Design review of the part built by this model. Coordinates are the model's own, in mm. A direction names the side the tool comes from. Coordinates: 2 decimals unless noted, no trailing zeros. Write each loop counter-clockwise with the first axis right and the second up, starting at its lowest first coordinate (ties: lowest second). Pieces come first, ordered by that corner, then holes.
Q1. Insertion check: pin 1 (3 mm diameter, centred on x = -8, z = 9, fed in from +Y); pin 2 (1.5 mm diameter, centred on x = 12, z = 9, fed in from -Y); pin 3 (3.5 mm diameter, centred on x = 3, z = 4.5, fed in from +Y). Each pin has a flat end and moves straight along its axis. Give the tip position at first contact, or say it passes through.
Q2. Machinability: for faces 5 (the flat face through (15, 10, 6)), 6 (the flat face through (0, -11, 6)), which of the approach directions +Z, -Z, +X, -X, +Y, -Y give a long, thin tool a straight path to every point of the face, cutting with its end or side? Answer none if there is none.
Q3. Take a section at C-C (z = 7.75). Give the boundary of the cut face in (x, y) (3 decimals), and give its area (3 significant figures).
Q4. Take a section at B-B (y = 14). Give the boundary of the cut face in (x, z).
Q5. Take a section at A-A (x = 0). Give the boundary of the cut face in (y, z) (3 decimals), and give its area (3 significant figures).
Q6. For probe 1 along Y at (x, z) = (0, 7.5) (3 decimals); probe 2 along X at (y, z) = (6, 5.5); probe 3 along X at (y, z) = (24, 2.75), list the stretches that pass through material, from the lowest coordinate up.
Q7. Mouldability with a two-part tool opening along Y and no side actions: class faces 1 (the flat face through (0, 11, 0)), 2 (the flat face through (-8.718, -2, 6)), 3 (the cylindrical face through (0, -40, 6)), 4 (the flat face through (0, 7, 6)) as pulls with the +Y half, pulls with the -Y half, needs draft (parallel to the pull), parting line crosses it, or undercut.
Q8. Take a section at D-D (x = 13.5). Give the boundary of the cut face in (y, z), and give its area (3 significant figures).
```python
from build123d import *

# Parameters (mm, degrees)
SKETCH1_R           = 9.625
SKETCH1_R_2         = 5
SKETCH1_W           = 18
SKETCH1_H           = 18
BOSS_EXTRUDE1_DEPTH = 12


with BuildPart() as part:
    # Sketch1 → Boss-Extrude1 (new body)
    with BuildSketch(Plane.XY):
        with BuildLine():
            Line((15, 45), (15, -25))
            ThreePointArc((15, -25), (0, -40), (-15, -25))
            Line((-15, -25), (-15, 45))
            ThreePointArc((-15, 45), (0, 60), (15, 45))
        make_face()
        with Locations((0, -25)):
            Circle(SKETCH1_R, mode=Mode.SUBTRACT)
        with Locations((0, 45)):
            Circle(SKETCH1_R_2, mode=Mode.SUBTRACT)
        with Locations((0, 21)):
            Rectangle(SKETCH1_W, SKETCH1_H, mode=Mode.SUBTRACT)
        with Locations((0.28234497, -2)):
            Rectangle(SKETCH1_W, SKETCH1_H, mode=Mode.SUBTRACT)
    extrude(amount=BOSS_EXTRUDE1_DEPTH)


solid = part.part
```
Response:
1. pin 1: stops at y = 58.52
1. pin 2: stops at y = -34.92
1. pin 3: stops at y = 59.95
2. face 5: +Z, -Z, +X, +Y, -Y
2. face 6: +Z, -Z
3. outline: (-15, -25) arc R15 ccw to (15, -25) - (15, 45) arc R15 ccw to (-15, 45) - close; hole circle Ø19.25 at (0, -25); hole (-9, 12) - (9, 12) - (9, 30) - (-9, 30) - close; hole (-8.718, -11) - (9.282, -11) - (9.282, 7) - (-8.718, 7) - close; hole circle Ø10 at (0, 45)
3. area: 1,790 mm2
4. outline: (-15, 0) - (-9, 0) - (-9, 12) - (-15, 12) - close; (9, 0) - (15, 0) - (15, 12) - (9, 12) - close
5. outline: (-40, 0) - (-34.625, 0) - (-34.625, 12) - (-40, 12) - close; (-15.375, 0) - (-11, 0) - (-11, 12) - (-15.375, 12) - close; (7, 0) - (12, 0) - (12, 12) - (7, 12) - close; (30, 0) - (40, 0) - (40, 12) - (30, 12) - close; (50, 0) - (60, 0) - (60, 12) - (50, 12) - close
5. area: 417 mm2
6. probe 1: y = -40 to -34.625, -15.375 to -11, 7 to 12, 30 to 40, 50 to 60
6. probe 2: x = -15 to -8.72, 9.28 to 15
6. probe 3: x = -15 to -9, 9 to 15
7. face 1: needs draft
7. face 2: undercut
7. face 3: pulls with the -Y half
7. face 4: undercut
8. outline: (-31.54, 0) - (51.54, 0) - (51.54, 12) - (-31.54, 12) - close
8. area: 997 mm2
